Answer from the drawing. Dimensions are ordinates in mm from the lowest x, y and z of the part. A direction names the side the tool comes from. Coordinates: 2 decimals unless noted, no trailing zeros. Loops run counter-clockwise (first coordinate to the right, second up) from the corner with the lowest first, then second, coordinate; pieces in that order, holes last.
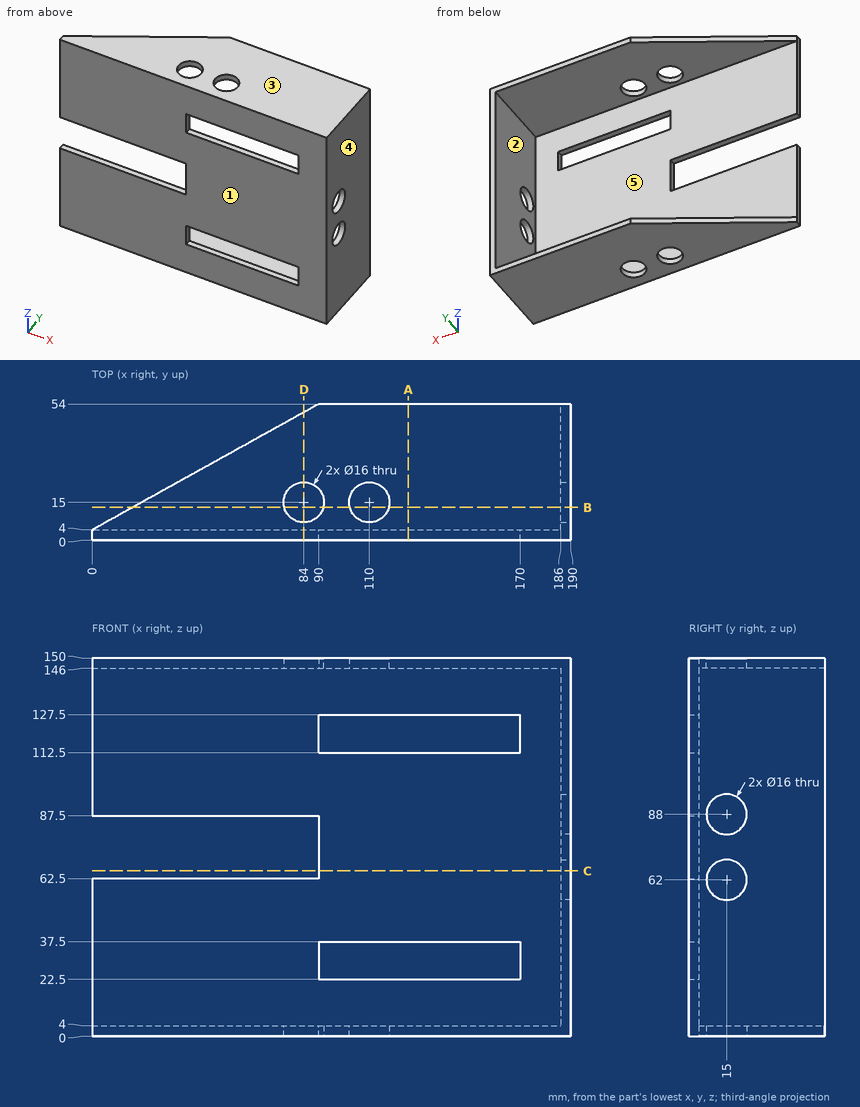
Item 1: A cutting plane is placed at B-B on y = 13. Give the number of separate pieces and of enclosed holes in the cut face, then the cut area to 3 significant figures.
Numbers:
separate pieces: 7
enclosed holes: 0
area: 1,590 mm2
Item 2: A cutting plane is placed at D-D on x = 84. Determine the outline of the cut face in (y, z).
Numbers:
outline: (0, 0) - (7, 0) - (7, 4) - (4, 4) - (4, 62.5) - (0, 62.5) - close; (0, 87.5) - (4, 87.5) - (4, 146) - (7, 146) - (7, 150) - (0, 150) - close; (23, 0) - (50.67, 0) - (50.67, 4) - (23, 4) - close; (23, 146) - (50.67, 146) - (50.67, 150) - (23, 150) - close
Item 3: Given pin 1 (25 mm diameter, centred on y = 39, z = 92.5, fed in from -X); pin 2 (1.2 mm diameter, centred on y = 1.5, z = 72, fed in from -X); pin 3 (12 mm diameter, centred on x = 134, z = 50.5, fed in from +Y), each flat-ended and moving along its own axis, determine where each tip first touches the part or whether it passes through.
Numbers:
pin 1: stops at x = 186
pin 2: stops at x = 90
pin 3: stops at y = 4
Item 4: A cutting plane is placed at C-C on z = 65.5. Determine the outline of the cut face in (x, y), then the cut area to 3 significant figures.
Numbers:
outline: (90, 0) - (190, 0) - (190, 7.81) - (186, 7.81) - (186, 4) - (90, 4) - close; (186, 22.19) - (190, 22.19) - (190, 54) - (186, 54) - close
area: 542 mm2
Item 5: Find the intervals of material crossed by line 1 along Z through (x, y) = (132, 3); line 2 along Y through (x, z) = (188.3, 88); line 3 along Z through (x, y) = (127.5, 27), in increasing order.
Numbers:
line 1: z = 0 to 22.5, 37.5 to 112.5, 127.5 to 150
line 2: y = 0 to 7, 23 to 54
line 3: z = 0 to 4, 146 to 150
Item 6: Determine the mould class of the marked faces 3, 4 and 5 for opening direction Z: released by +Z, released by -Z, zero draft, split by the parting line, or undercut.
Numbers:
face 3: released by +Z
face 4: zero draft
face 5: undercut
Item 7: Which of the six approach directions +Z, -Z, +X, -X, +Y, -Y give full straight-line access (tool end or side, diameter ignored) to the marked faces 1 and 2?
Numbers:
face 1: +Z, -Z, +X, -X, -Y
face 2: -X, +Y
Item 8: A cutting plane is placed at A-A on x = 125.5. Determine the outline of the cut face in (y, z), then the cut area to 3 significant figures.
Numbers:
outline: (0, 0) - (54, 0) - (54, 4) - (4, 4) - (4, 22.5) - (0, 22.5) - close; (0, 37.5) - (4, 37.5) - (4, 112.5) - (0, 112.5) - close; (0, 127.5) - (4, 127.5) - (4, 146) - (54, 146) - (54, 150) - (0, 150) - close
area: 880 mm2
